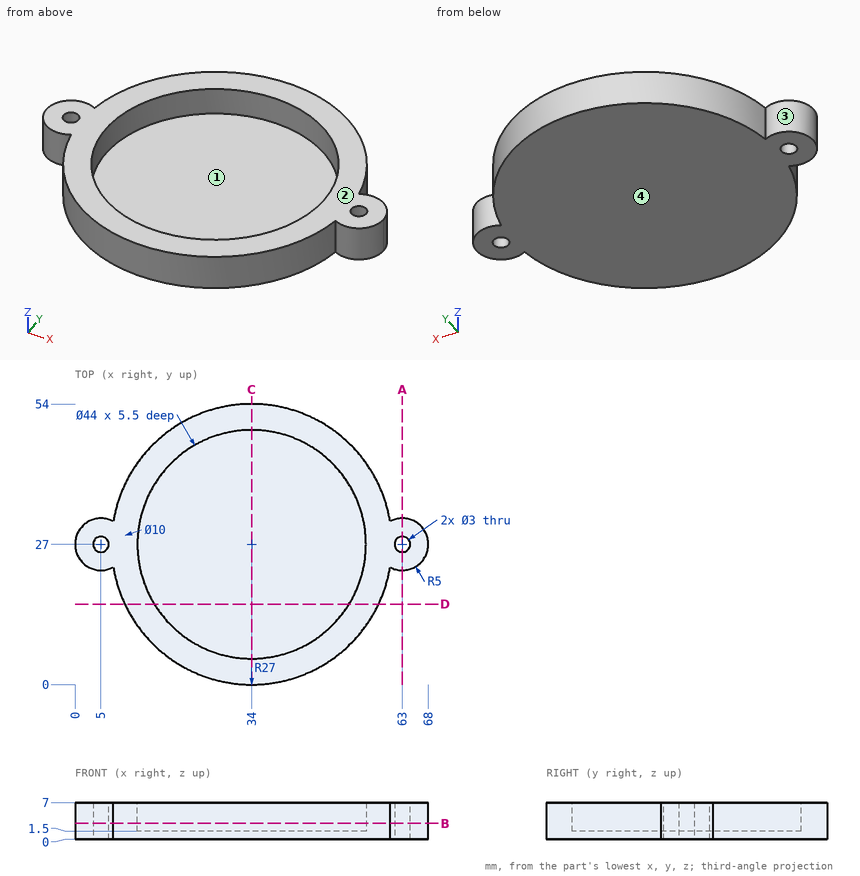
Geometry: see drawing. Coordinates: mm, zero at the bounding-box minimum. A direction names the side the tool comes from. Give positions to 0.01 mm unless a question says otherwise; leave off trailing zeros. Loops run counter-clockwise (first coordinate to the right, second up) from the corner with the lowest first, then second, coordinate; pieces in that order, holes last. Notation, with made-up numbers: (72, 69) -> (121, 69) arc R18 ccw to (121, 76) -> close; hole circle Ø1 at (-1, 87). An arc over 180 degrees is marked (long way). Answer as a JSON object with one key per item and string values. Group by question number.
Item 1: Line query: probe 1 along Y at (x, z) = (34, 3.25); probe 2 along Z at (x, y) = (20, 33.5); probe 3 along Y at (x, z) = (30, 5.75). Output: solid intervals per line, ascending.
Item 2: Cut plane D-D, the plane y = 15.5. Return the cut outline in (x, z) (3 decimals).
Item 3: Reachability of the marked faces 1 and 2 from +Z, -Z, +X, -X, +Y, -Y: full face, straight path, thin tool, end or side. Return the list, or none.
Item 4: Pull-direction query (X, two-part tool) for the marked faces 3 and 4; classes: released by +X, released by -X, zero draft, split by the parting line, or undercut.
Item 5: Cut plane B-B, the plane z = 3. Return the cut outline in (x, y).
Item 6: Pin query (flat end, axial travel): P1, Ø1.5, axis at x = 53.5, z = 3.5, coming from the +Y side; P2, Ø6, axis at x = 30.5, y = 23, coming from the +Z side; P3, Ø3, axis at x = 36.5, z = 3, coming from the +Y side; P4, Ø2.5, axis at x = 5, y = 27, coming from the -Z side. Return the tip coordinate at first contact, or that it passes through.
Item 7: Cut plane A-A, the plane x = 63. Return the cut outline in (y, z).
Item 8: Cut plane C-C, the plane x = 34. Return the cut outline in (y, z).
Checks:
{
 "1": {"probe 1": "y = 0 to 5, 49 to 54", "probe 2": "z = 0 to 1.5", "probe 3": "y = 0.3 to 5.37, 48.63 to 53.7"},
 "2": {"outline": "(9.572, 0) -> (58.428, 0) -> (58.428, 7) -> (52.755, 7) -> (52.755, 1.5) -> (15.245, 1.5) -> (15.245, 7) -> (9.572, 7) -> close"},
 "3": {"face 1": "+Z", "face 2": "+Z, +X, -X, +Y, -Y"},
 "4": {"face 3": "undercut", "face 4": "zero draft"},
 "5": {"outline": "(7.36, 22.59) arc R27 ccw to (60.64, 22.59) arc R5 ccw (long way) to (60.64, 31.41) arc R27 ccw to (7.36, 31.41) arc R5 ccw (long way) to start; hole circle Ø3 at (5, 27); hole circle Ø44 at (34, 27); hole circle Ø3 at (63, 27)"},
 "6": {"P1": "stops at y = 46.43", "P2": "stops at z = 1.5", "P3": "stops at y = 53.98", "P4": "passes through"},
 "7": {"outline": "(22, 0) -> (25.5, 0) -> (25.5, 7) -> (22, 7) -> close; (28.5, 0) -> (32, 0) -> (32, 7) -> (28.5, 7) -> close"},
 "8": {"outline": "(0, 0) -> (54, 0) -> (54, 7) -> (49, 7) -> (49, 1.5) -> (5, 1.5) -> (5, 7) -> (0, 7) -> close"}
}
